Build history of the part. All positions in model axes, mm. Give positions to 0.01 mm unless a question says otherwise; leave off trailing zeros. Order: outer loops, then holes, each group sorted by start corner. A loop starts at its lowest first (then second) coordinate and runs counter-clockwise, first axis right, second up. Notation, with made-up numbers: (-17, -31) -> (10, -31) arc R30 cw to (10, 8) -> close; hole circle Ø3 at (-13, -17.75). An arc over 180 degrees is marked (long way). One line per question, with ' | ' between items. Start each with the question number.
(1) Drill centre lines: L1, parallel to Z at x = 78.5, y = -380; L2, parallel to Z at x = 67.5, y = -134; L3, parallel to X at y = 2, z = 80. Where is each one in solid material? Low to high. Write a range as from..to.
(2) Cut at D-D (z = 6). Give the cut face in (x, y), then the cut area to 3 significant figures.
(3) Cut at A-A (x = 65.5). Give the cut face in (y, z).
(4) Cut at B-B (z = 69.5). Give the cut face in (x, y), then the cut area to 3 significant figures.
(5) Pin check, flat tips, straight feed: pin 1 Ø10 at (y, z) = (-955, 84) entering from +X; pin 2 Ø8 at (y, z) = (-311.5, 82.5) entering from -X; pin 3 Ø2 at (x, z) = (79.5, 42) entering from -Y. Stop position of each tip, or through.
(6) Cut at C-C (y = -260). Give the cut face in (x, z), then the cut area to 3 significant figures.
from build123d import *

# Parameters (mm, degrees)
F1_DEPTH = 127
F2_W     = 111.76
F2_H     = 50.8
F3_DEPTH = 12.7
F5_DEPTH = 138.684


with BuildPart() as f1:
    # F0 (on Right) → F1 (new body)
    with BuildSketch(Plane.YZ):
        Polygon((66.087551, 104.79458), (-949.912449, 104.79458), (-949.912449, 41.29458), (-861.012449, -22.20542), (-492.712449, -22.20542), (66.087551, 79.39458), align=None)
    extrude(amount=F1_DEPTH)

    # F2 (on face) → F3 (join)
    with BuildSketch(Plane.XZ.offset(949.912449)):
        with Locations((63.28021, 73.04458)):
            Rectangle(F2_W, F2_H)
    extrude(amount=F3_DEPTH)

    # F4 (on face) → F5 (cut)
    with BuildSketch(Plane.XY.offset(104.79458)):
        Polygon((0, -492.712449), (50.8, 66.087551), (0, 66.087551), align=None)
        Polygon((127, 66.087551), (76.2, 66.087551), (127, -492.712449), align=None)
    extrude(amount=-F5_DEPTH, mode=Mode.SUBTRACT)


solid = f1.part
Result set:
1) L1: z = -1.71..104.79 | L2: z = 43.02..104.79 | L3: x = 44.97..82.03
2) outline: (0, -900.5) -> (127, -900.5) -> (127, -492.71) -> (112.9, -337.58) -> (14.1, -337.58) -> (0, -492.71) -> close | area: 69,300 mm2
3) outline: (-962.61, 47.64) -> (-949.91, 47.64) -> (-949.91, 41.29) -> (-861.01, -22.21) -> (-492.71, -22.21) -> (66.09, 79.39) -> (66.09, 104.79) -> (-949.91, 104.79) -> (-949.91, 98.44) -> (-962.61, 98.44) -> close
4) outline: (0, -949.91) -> (7.4, -949.91) -> (7.4, -962.61) -> (119.16, -962.61) -> (119.16, -949.91) -> (127, -949.91) -> (127, -492.71) -> (81.15, 11.67) -> (45.85, 11.67) -> (0, -492.71) -> close | area: 100,000 mm2
5) pin 1: stops at x = 119.16 | pin 2: stops at x = 16.11 | pin 3: stops at y = -949.91
6) outline: (21.16, 20.11) -> (105.84, 20.11) -> (105.84, 104.79) -> (21.16, 104.79) -> close | area: 7,170 mm2
